Build history of the part. All positions in model axes, mm. Give positions to 0.01 mm unless a question says otherwise; leave off trailing zeros. Order: outer loops, then holes, each group sorted by start corner. A loop starts at its lowest first (then second) coordinate and runs counter-clockwise, first axis right, second up. Notation, with made-up numbers: (-21.5, -19) -> (-2.5, -19) arc R19 cw to (-2.5, -14) -> close; hole circle Ø8 at (64.25, 44.5). An arc over 180 degrees is marked (long way). One line per question, with ' | ' between items. Start each with the question number.
(1) Cut at B-B (x = -2.75). Give the cut face in (y, z), then the cut area to 3 significant figures.
(2) Cut at C-C (z = 3). Give the cut face in (x, y), then the cut area to 3 significant figures.
(3) Cut at A-A (y = -16). Give the cut face in (x, z).
(4) Pull direction Y, two halves, no side cores. Call faces 1 (the face through (-12, 76.2, 25)), 2 (the face through (0, 63, 24)), 3 (the face through (-12, 50.8, 31)): +Y half, -Y half, draft (parallel to the pull), parting line (faces both ways), or undercut.
(5) Pin check, flat tips, straight feed: pin 1 Ø4 at (x, y) = (-11.5, 42) entering from +Z; pin 2 Ø1.5 at (x, y) = (-13, 56.5) entering from -Z; pin 3 Ø4 at (x, y) = (-6.5, 36.5) entering from +Z. Stop position of each tip, or through.
(6) Cut at D-D (y = 8.5). Give the cut face in (x, z).
(7) Drill centre lines: L1, parallel to Z at x = -12, y = -20; L2, parallel to Y at x = -2, z = 49; L3, parallel to Z at x = -8, y = -21. Where is each one in solid material? Low to high. Write a range as from..to.
from build123d import *

# Parameters (mm, degrees)
F0_R     = 6.076519
F1_DEPTH = 25.4
F2_DEPTH = 25.4


with BuildPart() as f1:
    # F0 (on Front) → F1 (new body)
    with BuildSketch(Plane.XZ):
        with BuildLine():
            ThreePointArc((0, 0), (-11.868954, 11.868954), (-23.737907, 0))
            ThreePointArc((-23.737907, 0), (-11.868954, -11.868954), (0, 0))
        make_face()
        with Locations((-11.868954, 0)):
            Circle(F0_R, mode=Mode.SUBTRACT)
        with BuildLine():
            Line((-23.737907, 48.319295), (-23.737907, 0))
            ThreePointArc((-23.737907, 0), (-11.868954, 11.868954), (0, 0))
            Line((0, 0), (0, 48.319295))
            ThreePointArc((0, 48.319295), (-11.868954, 60.188249), (-23.737907, 48.319295))
        make_face()
        with Locations((-11.868954, 48.319295)):
            Circle(F0_R, mode=Mode.SUBTRACT)
    extrude(amount=F1_DEPTH)

    # F0 (on Front) → F2 (join)
    with BuildSketch(Plane.XZ):
        with BuildLine():
            ThreePointArc((0, 0), (-11.868954, 11.868954), (-23.737907, 0))
            ThreePointArc((-23.737907, 0), (-11.868954, -11.868954), (0, 0))
        make_face()
        with Locations((-11.868954, 0)):
            Circle(F0_R, mode=Mode.SUBTRACT)
    extrude(amount=-F2_DEPTH)

    # F3: F1 across face


with BuildPart() as f1_1:
    add(f1.part)
    add(f1.part.mirror(Plane(origin=(-11.868954, 25.4, 0), x_dir=(1, 0, 0), z_dir=(0, 1, 0))))


solid = f1_1.part
Result set:
1) outline: (-25.4, -7.6) -> (76.2, -7.6) -> (76.2, 55.92) -> (50.8, 55.92) -> (50.8, 7.6) -> (0, 7.6) -> (0, 55.92) -> (-25.4, 55.92) -> close | area: 4,000 mm2
2) outline: (-23.74, -25.4) -> (-17.15, -25.4) -> (-17.15, 76.2) -> (-23.74, 76.2) -> (-23.74, 50.8) -> (-23.35, 50.8) -> (-23.35, 0) -> (-23.74, 0) -> close; (-6.58, -25.4) -> (0, -25.4) -> (0, 0) -> (-0.39, 0) -> (-0.39, 50.8) -> (0, 50.8) -> (0, 76.2) -> (-6.58, 76.2) -> close | area: 1,300 mm2
3) outline: (-23.74, 0) arc R11.87 ccw to (0, 0) -> (0, 48.32) arc R11.87 ccw to (-23.74, 48.32) -> close; hole circle Ø12.15 at (-11.87, 0); hole circle Ø12.15 at (-11.87, 48.32)
4) face 1: +Y half | face 2: draft | face 3: undercut
5) pin 1: stops at z = 11.87 | pin 2: stops at z = -11.86 | pin 3: stops at z = 11.38
6) outline: (-23.74, 0) arc R11.87 ccw to (0, 0) arc R11.87 ccw to start; hole circle Ø12.15 at (-11.87, 0)
7) L1: z = -11.87..-6.08, 6.08..42.24, 54.39..60.19 | L2: y = -25.4..0, 50.8..76.2 | L3: z = -11.22..-4.69, 4.69..43.63, 53..59.54
